The figure shows three views and two pictorial views of one solid part (mm, origin at its lowest corner). Answer the questions. Round coordinates to 2 decimals unless told otherwise and drop trailing zeros. Order: outer loops, then holes, each group sorted by start corner. A loop starts at its lowest first (then second) coordinate and runs counter-clockwise, first axis right, second up. Notation, with made-up numbers: (60.5, 62) -> (94.5, 62) arc R17 cw to (94.5, 86) -> close; hole circle Ø8 at (54, -24.5). An arc over 180 degrees is marked (long way). One line per item, written item: value. Start each with the question number.
1. Flat-ended cylindrical pins translate along their axes: pin 1 Ø4 at (x, y) = (11, 62) entering from -Z; pin 2 Ø8 at (x, z) = (7, 65.5) entering from +Y; pin 3 Ø2 at (x, z) = (12.5, 221) entering from +Y. Find the tip coordinate at first contact, or state that the pin passes through.
2. Section A-A (x = 2.75) is taken. Give the vertices of the cut face in (y, z).
3. Section C-C (z = 204.5) is taken. Give the vertices of the cut face in (x, y).
4. Consider line 1 (Y direction, x = 9.25, z = 93); line 2 (Y direction, x = 6.5, z = 184); line 3 (Z direction, x = 6.5, y = 213.5). Determine where each line is inside the solid, lowest interval first.
5. Section B-B (y = 65.5) is taken. Give the vertices of the cut face in (x, z).
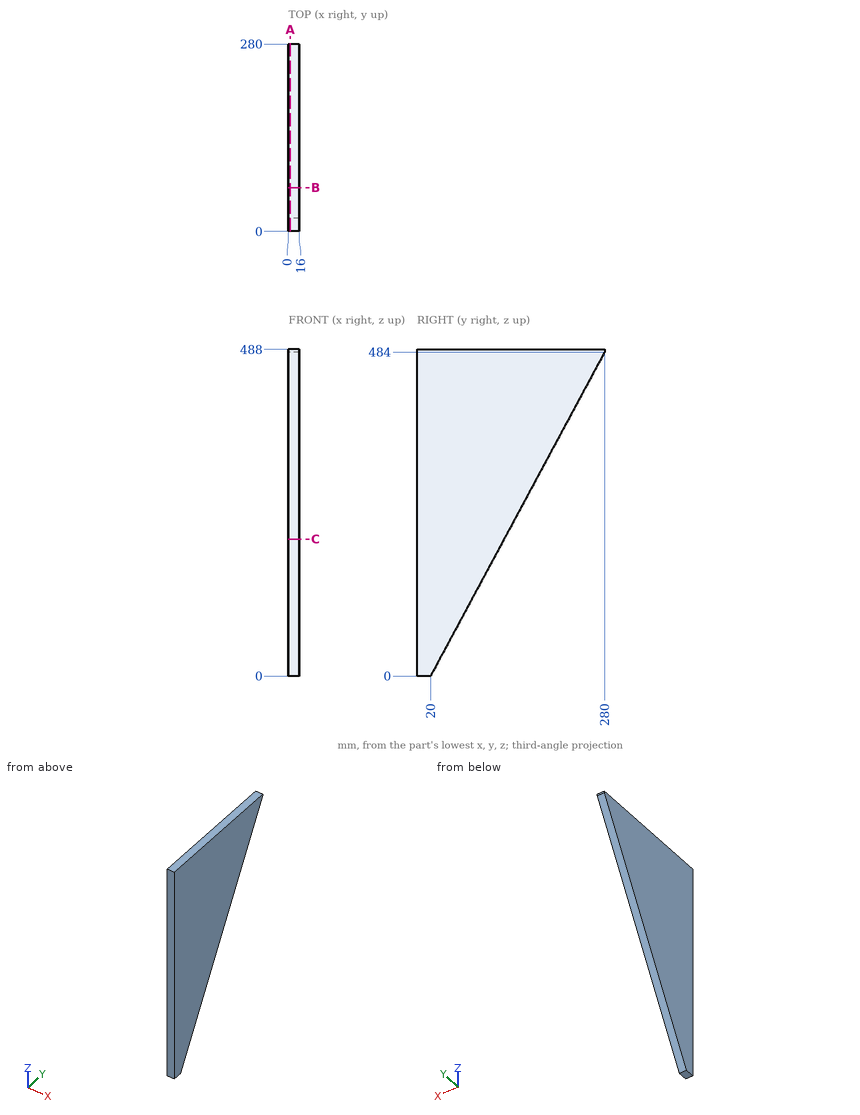
Answer:
1. pin 1: z = 74.46
1. pin 2: y = 57.33
1. pin 3: y = 139.26
2. outline: (0, 0) -> (20, 0) -> (280, 484) -> (280, 488) -> (0, 488) -> close
3. outline: (0, 0) -> (16, 0) -> (16, 129.86) -> (0, 129.86) -> close
4. line 1: 0 to 69.96
4. line 2: 0 to 118.84
4. line 3: 360.21 to 488
5. outline: (0, 84.7) -> (16, 84.7) -> (16, 488) -> (0, 488) -> close
